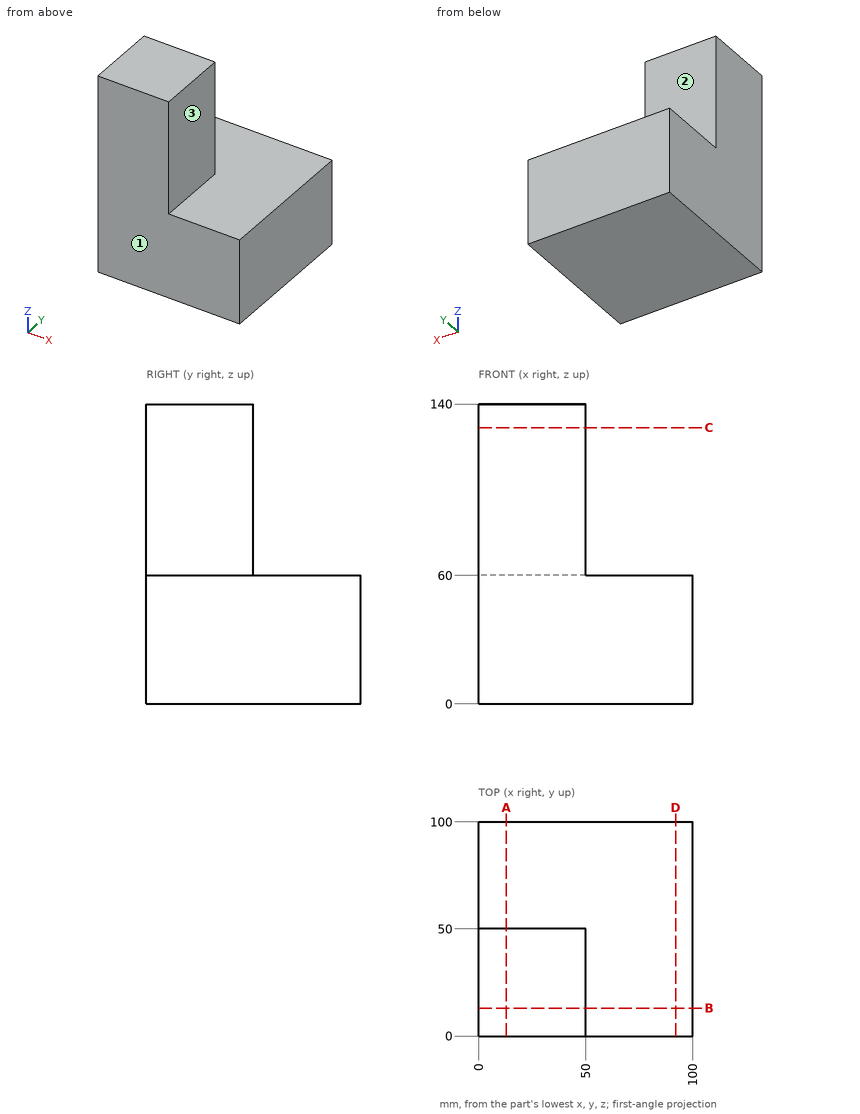
Here's the drawing with two shaded views (mm, measured from the low corner). I have some questions. A direction names the side the tool comes from. Coordinates: 2 decimals unless noted, no trailing zeros. Loops run counter-clockwise (first coordinate to the right, second up) from the corner with the lowest first, then second, coordinate; pieces in that order, holes last. Notation, with made-up numbers: (-26, 4.25) -> (15, 4.25) arc R35 ccw to (15, 43.25) -> close; hole circle Ø8 at (-5.75, 2.25). An arc over 180 degrees is marked (long way). Put each result on its own line as item: value. Start each with the question number.
Q1. I want a section at A-A (x = 13). Write out the boundary of the cut face in (y, z), plus the area to 3 significant figures.
Q2. I'm going to push flat-ended pins straight in: P1, Ø25, axis at y = 29.5, z = 98.5, coming from the +X side; P2, Ø12, axis at x = 60.5, y = 88.5, coming from the +Z side. Where does each tip first touch, or does it pass through?
Q3. I want a section at C-C (z = 129). Write out the boundary of the cut face in (x, y).
Q4. I want a section at D-D (x = 92). Write out the boundary of the cut face in (y, z), plus the area to 3 significant figures.
Q5. If I drill on line 1 (X direction, y = 28.5, z = 110); line 2 (Z direction, x = 93.5, y = 81), over which ranges is the centre line in solid material (lowest first)? Write a range as [from, to].
Q6. For the marked faces 1, 2 and 3, which set-ups out of +Z, -Z, +X, -X, +Y, -Y let a thin tool reach every point of the face, with its end or its side?
Taken from the geometry:
1. outline: (0, 0) -> (100, 0) -> (100, 60) -> (50, 60) -> (50, 140) -> (0, 140) -> close
1. area: 10,000 mm2
2. P1: stops at x = 50
2. P2: stops at z = 60
3. outline: (0, 0) -> (50, 0) -> (50, 50) -> (0, 50) -> close
4. outline: (0, 0) -> (100, 0) -> (100, 60) -> (0, 60) -> close
4. area: 6,000 mm2
5. line 1: x = [0, 50]
5. line 2: z = [0, 60]
6. face 1: +Z, -Z, +X, -X, -Y
6. face 2: +Z, +X, -X, +Y
6. face 3: +Z, +X, +Y, -Y
